Design review of the part built by this model. Coordinates are the model's own, in mm. A direction names the side the tool comes from. Coordinates: 2 decimals unless noted, no trailing zeros. Write each loop counter-clockwise with the first axis right and the second up, starting at its lowest first coordinate (ties: lowest second). Pieces come first, ordered by that corner, then holes. Notation, with made-up numbers: (15, 4) - (71, 4) arc R12 ccw to (71, 16) - close; hole circle Ø5 at (-20, 73.5). An arc over 180 degrees is marked (long way). Answer as a JSON object with one key per item and string values.
```python
from build123d import *

# Parameters (mm, degrees)
SKICA2_W                = 6
SKICA2_H                = 42
SKICA2_R                = 1.35
SKICA2_H_2              = 25
P_IDAT_VYSUNUT_M1_DEPTH = 2.5
SKICA3_W                = 6
SKICA3_H                = 8
P_IDAT_VYSUNUT_M2_DEPTH = 2.5
ZAOBLIT1_R              = 10
ZAOBLIT2_R              = 1


with BuildPart() as part:
    # Skica2 → Přidat vysunutím1 (new body)
    # profile 1 of 2: a face of its own
    with BuildSketch(Plane.XY):
        with Locations((-3, -21)):
            Rectangle(SKICA2_W, SKICA2_H)
        with Locations((-3, -38.83625)):
            Circle(SKICA2_R, mode=Mode.SUBTRACT)
        with Locations((-3, -3.16375)):
            Circle(SKICA2_R, mode=Mode.SUBTRACT)
    # profile 2 of 2: a face of its own
    with BuildSketch(Plane.XY):
        with Locations((-3, -54.5)):
            Rectangle(SKICA2_W, SKICA2_H_2)
    extrude(amount=P_IDAT_VYSUNUT_M1_DEPTH)

    # Skica3 → Přidat vysunutím2 (add)
    with BuildSketch(Plane.XZ.offset(67)):
        with Locations((-3, 4)):
            Rectangle(SKICA3_W, SKICA3_H)
    extrude(amount=-P_IDAT_VYSUNUT_M2_DEPTH)

    # Zaoblit1
    # the kernel refuses this fillet: 10 mm, written as the material it adds along each edge
    with BuildSketch(Plane(origin=(0, -64.5, 2.5), x_dir=(0, 1, 0), z_dir=(-1, 0, 0))) as zaoblit1_piece_1:
        with BuildLine():
            CenterArc((8.93028555, -10), ZAOBLIT1_R, 90, 63.25631605)
            Line((0, -5.5), (-0.178605711, -5.41))
            ThreePointArc((-0.178605711, -5.41), (-0.2, -2.75), (-0.2, 0))
            Line((-0.2, 0), (0, 0.2))
            Line((0, 0.2), (8.93028555, 0.2))
            Line((8.93028555, 0.2), (8.93028555, 0))
        make_face()
    extrude(amount=6)

    # Zaoblit2
    zaoblit2_edges = [part.edges().sort_by_distance(p)[0] for p in [
        (-3, -64.5, 8),
    ]]
    fillet(zaoblit2_edges, radius=ZAOBLIT2_R)


solid = part.part
```
(1) To check wall thickness, follow line 1 (Y direction, x = -3, z = 1.55); line 2 (Z direction, x = -0.7, y = -27); line 3 (Y direction, x = -2.05, z = 1.25). State the ranges of each line that lie inside material, in increasing order. Write a range as from..to.
Solved:
{"line 1": "y = -67..-40.19, -37.49..-4.51, -1.81..0", "line 2": "z = 0..2.5", "line 3": "y = -67..-39.8, -37.88..-4.12, -2.2..0"}
(2) Tool access review of faces 1 (the face through (-3, -27, 2.5)), 2 (the face through (-6, -33, 1)): name each direction out of +Z, -Z, +X, -X, +Y, -Y from which nothing blocks a thin tool from reaching the whole face with its end or side.
Solved:
{"face 1": "+Z, +X, -X, +Y", "face 2": "+Z, -Z, -X, +Y, -Y"}
(3) For pin 1 (1.6 mm diameter, centred on x = -3, y = -38.84, fed in from +Z); pin 2 (3 mm diameter, centred on x = -3.5, z = 5, fed in from +Y); pin 3 (1.5 mm diameter, centred on x = -3.5, y = -7.5, fed in from +Z), all flat-tipped, find the tip position at first contact; note any pin that passes through.
Solved:
{"pin 1": "passes through", "pin 2": "stops at y = -59.93", "pin 3": "stops at z = 2.5"}
(4) Take a section at C-C, the plane z = 4.5. Write out the cut boundary in (x, y), and give its area (3 significant figures).
Solved:
{"outline": "(-6, -67) - (0, -67) - (0, -61.57) - (-6, -61.57) - close", "area": "32.6 mm^2"}
(5) The part is to be moulded in two halves that separate along X. For faces 3 (the face through (0, -33, 1)), 4 (the face through (-1.7, -2.8, 1.2)), 5 (the face through (-3, 0, 1)), say which applies: pulls with the +X half, pulls with the -X half, needs draft (parallel to the pull), parting line crosses it, or undercut.
Solved:
{"face 3": "pulls with the +X half", "face 4": "undercut", "face 5": "needs draft"}
(6) Take a section at B-B, the plane y = -14.5. Write out the cut boundary in (x, z), and give its area (3 significant figures).
Solved:
{"outline": "(-6, 0) - (0, 0) - (0, 2.5) - (-6, 2.5) - close", "area": "15.0 mm^2"}
(7) Take a section at A-A, the plane x = -3. Write out the cut boundary in (y, z).
Solved:
{"outline": "(-67, 0) - (-40.19, 0) - (-40.19, 2.5) - (-55.57, 2.5) arc R10 cw to (-64.23, 7.5) arc R1 ccw to (-65.1, 8) - (-67, 8) - close; (-37.49, 0) - (-4.51, 0) - (-4.51, 2.5) - (-37.49, 2.5) - close; (-1.81, 0) - (0, 0) - (0, 2.5) - (-1.81, 2.5) - close"}
